Drawing for the job (mm, zero at the part's lowest x, y, z). A direction names the side the tool comes from. Coordinates: 2 decimals unless noted, no trailing zeros. Write each loop counter-clockwise with the first axis right and the second up, starting at its lowest first coordinate (ties: lowest second). Pieces come first, ordered by that corner, then holes. Notation, with made-up numbers: (65.5, -4) -> (79.5, -4) arc R20 cw to (79.5, 27) -> close; hole circle Ø3 at (35.5, 56.5). An arc over 180 degrees is marked (long way). Write item = value, one per line. Start each with the question number.
Q1. Band-saw the part on C-C, the plane x = 82.5. List the corners of the cut face in (y, z), plus the area to 3 significant figures.
Q2. Band-saw the part on A-A, the plane z = 26. List the corners of the cut face in (x, y).
Q3. Pin check, flat tips, straight feed: P1, Ø10, axis at x = 23.495, y = 71.755, coming from the +Z side; P2, Ø3, axis at y = 12.5, z = 66, coming from the +X side; P3, Ø10, axis at x = 46, y = 37.5, coming from the -Z side; P4, Ø8, axis at x = 186.055, y = 71.755, coming from the -Z side. Stop position of each tip, or through.
Q4. Pull direction X, two halves, no side cores. Call the marked faces 1, 2 and 3: released by +X, released by -X, zero draft, split by the parting line, or undercut.
Q5. Probe line 1 (X direction, y = 18, z = 9.5); line 2 (Z direction, x = 49.5, y = 67.5); line 3 (Z direction, x = 113, y = 41.5). List the from-to ranges inside material, lowest first.
Q6. Tool access for the marked faces 4, 5, 6, 7 and 8: list every direction of +Z, -Z, +X, -X, +Y, -Y with a clear straight run to the whole face (end or side of a thin tool).
Q7. Band-saw the part on B-B, the plane y = 38. List the corners of the cut face in (x, z).
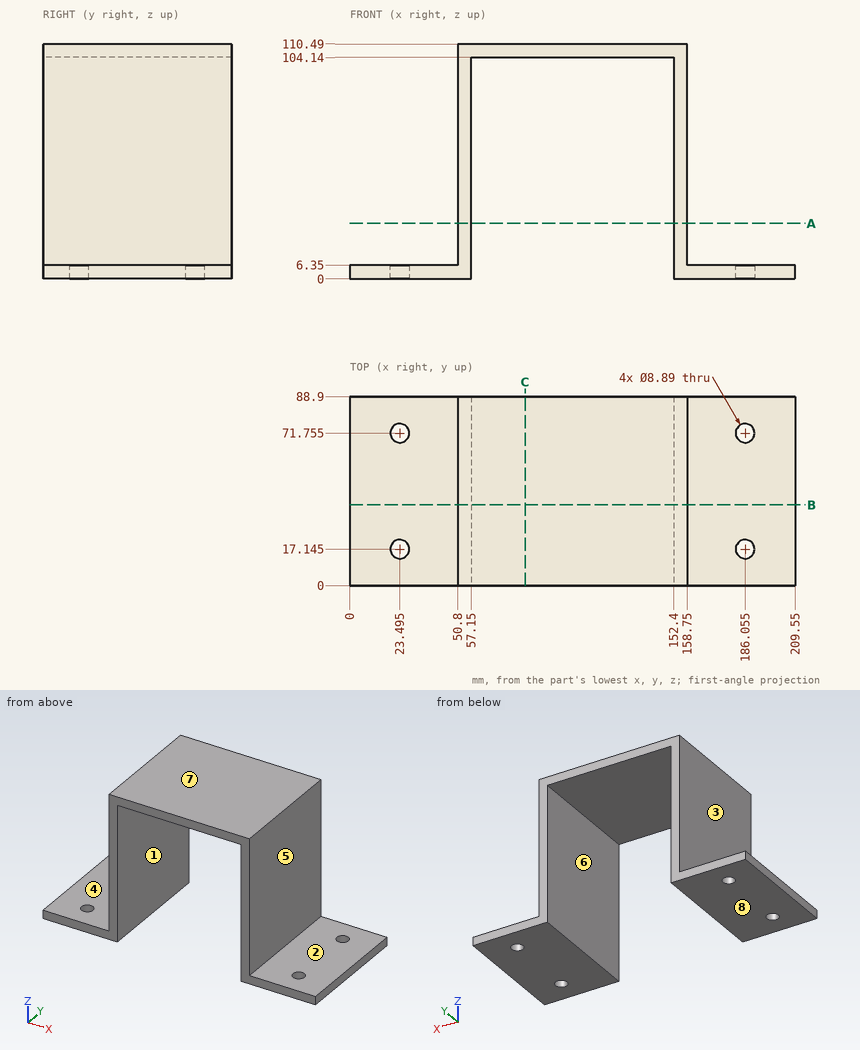
Ans:
q1.outline = (0, 104.14) -> (88.9, 104.14) -> (88.9, 110.49) -> (0, 110.49) -> close
q1.area = 565 mm2
q2.outline = (50.8, 0) -> (57.15, 0) -> (57.15, 88.9) -> (50.8, 88.9) -> close; (152.4, 0) -> (158.75, 0) -> (158.75, 88.9) -> (152.4, 88.9) -> close
q3.P1 = 6.35
q3.P2 = 158.75
q3.P3 = 0
q3.P4 = through
q4.face_1 = undercut
q4.face_2 = zero draft
q4.face_3 = released by -X
q5.line_1 = 50.8 to 57.15, 152.4 to 158.75
q5.line_2 = 0 to 6.35
q5.line_3 = 104.14 to 110.49
q6.face_4 = +Z, -X, +Y, -Y
q6.face_5 = +Z, +X, +Y, -Y
q6.face_6 = -Z, +Y, -Y
q6.face_7 = +Z, +X, -X, +Y, -Y
q6.face_8 = -Z, +X, -X, +Y, -Y
q7.outline = (0, 0) -> (57.15, 0) -> (57.15, 104.14) -> (152.4, 104.14) -> (152.4, 0) -> (209.55, 0) -> (209.55, 6.35) -> (158.75, 6.35) -> (158.75, 110.49) -> (50.8, 110.49) -> (50.8, 6.35) -> (0, 6.35) -> close
